Could you check a few things on this model? Use its own coordinates, in mm. A direction names the side the tool comes from. Coordinates: 2 decimals unless noted, no trailing zeros. Loops run counter-clockwise (first coordinate to the right, second up) from the corner with the lowest first, then second, coordinate; pieces in that order, holes last.
Autodesk Inventor part; units mm, degrees
ref_plane "Work Plane1" through (-19.708, -8.44, -77.2303) normal (0, 1, 0) x (0, 0, 1)
ref_plane "YZ Plane" through (0, 0, 0) normal (1, 0, 0) x (0, 1, 0)
ref_plane "XZ Plane" through (0, 0, 0) normal (0, 1, 0) x (-1, 0, 0)
sketch "Sketch1" plane through (0, 0, 0) normal (0, 1, 0) x (-1, 0, 0)
  line L0 (7.5, 17.125) -> (-7.5, 17.125)
  line L1 (-9.5, 15.125) -> (-9.5, -15.125)
  line L2 (-7.5, -17.125) -> (7.5, -17.125)
  line L3 (9.5, -15.125) -> (9.5, 15.125)
  line L4 (9.5, 17.125) -> (-9.5, -17.125) construction
  line L5 (-9.5, 17.125) -> (9.5, -17.125) construction
  arc A0 (7.5, -17.125) -> (9.5, -15.125) centre (7.5, -15.125) ccw
  arc A1 (-9.5, -15.125) -> (-7.5, -17.125) centre (-7.5, -15.125) ccw
  arc A2 (-7.5, 17.125) -> (-9.5, 15.125) centre (-7.5, 15.125) ccw
  arc A3 (9.5, 15.125) -> (7.5, 17.125) centre (7.5, 15.125) ccw
  point P0 (0, 0)
  dimension "d0" = 19
  dimension "d1" = 34.25
  dimension "d2" = 2
extrude "Extrusion1" add sketch "Sketch1" along normal blind 1.28
sketch "Sketch2" plane through (0, 1.28, 0) normal (0, 1, 0) x (1, 0, 0)
  line L0 (8.5, -12.175) -> (8.5, 15.825)
  line L1 (8.5, 15.825) -> (-8.5, 15.825)
  line L2 (-8.5, 15.825) -> (-8.5, -12.175)
  line L3 (-8.5, -12.175) -> (8.5, 15.825) construction
  line L4 (8.5, -12.175) -> (-8.5, 15.825) construction
  line L5 (7.5, 17.125) -> (-7.5, 17.125)
  line L6 (0, 17.125) -> (0, 15.825)
  line L7 (-6, -10.975) -> (6, -10.975)
  line L8 (6, -10.975) -> (6, -12.175)
  line L9 (-6, -12.175) -> (-6, -10.975)
  line L10 (-8.5, -12.175) -> (-6, -12.175)
  line L11 (6, -12.175) -> (8.5, -12.175)
  point P0 (0, 0)
  point P1 (0, 15.825)
  dimension "d5" = 17
  dimension "d6" = 28
  dimension "d7" = 1.3
  dimension "d9" = 1.2
extrude "Extrusion2" add sketch "Sketch2" along normal blind 1.28
sketch "Sketch3" plane through (0, 0, 0) normal (0, -1, 0) x (1, 0, 0)
  line L0 (5.75, -9.895) -> (-5.75, -9.895)
  line L1 (-5.75, -9.895) -> (-5.75, 6.605)
  line L2 (-5.75, 6.605) -> (5.75, 6.605)
  line L3 (5.75, 6.605) -> (5.75, -9.895)
  line L4 (7.5, -17.125) -> (-7.5, -17.125)
  line L5 (0, -17.125) -> (0, -9.895)
  point P0 (0, 0)
  point P1 (0, -9.895)
  dimension "d12" = 11.5
  dimension "d13" = 16.5
  dimension "d14" = 7.23
extrude "Extrusion3" add sketch "Sketch3" along normal blind 1.28
sketch "Sketch4" plane through (0, 0, 0) normal (0, -1, 0) x (1, 0, 0)
  line L0 (-7.5, 17.125) -> (7.5, 17.125)
  line L1 (0, 17.125) -> (0, 15.125)
  line L2 (0.2, 15.125) -> (2.24, 15.125)
  line L3 (2.44, 14.925) -> (2.44, 12.885)
  line L4 (2.24, 12.685) -> (0.2, 12.685)
  line L5 (0, 12.885) -> (0, 14.925)
  line L6 (0, 14.925) -> (0.2, 15.125)
  line L7 (2.24, 15.125) -> (2.44, 14.925)
  line L8 (2.44, 12.885) -> (2.24, 12.685)
  line L9 (0.2, 12.685) -> (0, 12.885)
  line L10 (2.64, 15.125) -> (4.68, 15.125)
  line L11 (4.88, 14.925) -> (4.88, 12.885)
  line L12 (4.68, 12.685) -> (2.64, 12.685)
  line L13 (2.44, 12.885) -> (2.44, 14.925)
  line L14 (2.44, 14.925) -> (2.64, 15.125)
  line L15 (4.68, 15.125) -> (4.88, 14.925)
  line L16 (4.88, 12.885) -> (4.68, 12.685)
  line L17 (2.64, 12.685) -> (2.44, 12.885)
  line L18 (5.08, 15.125) -> (7.12, 15.125)
  line L19 (7.32, 14.925) -> (7.32, 12.885)
  line L20 (7.12, 12.685) -> (5.08, 12.685)
  line L21 (4.88, 12.885) -> (4.88, 14.925)
  line L22 (4.88, 14.925) -> (5.08, 15.125)
  line L23 (7.12, 15.125) -> (7.32, 14.925)
  line L24 (7.32, 12.885) -> (7.12, 12.685)
  line L25 (5.08, 12.685) -> (4.88, 12.885)
  line L26 (-2.24, 15.125) -> (-0.2, 15.125)
  line L27 (0, 14.925) -> (0, 12.885)
  line L28 (-0.2, 12.685) -> (-2.24, 12.685)
  line L29 (-2.44, 12.885) -> (-2.44, 14.925)
  line L30 (-2.44, 14.925) -> (-2.24, 15.125)
  line L31 (-0.2, 15.125) -> (0, 14.925)
  line L32 (0, 12.885) -> (-0.2, 12.685)
  line L33 (-2.24, 12.685) -> (-2.44, 12.885)
  line L34 (-4.68, 15.125) -> (-2.64, 15.125)
  line L35 (-2.44, 14.925) -> (-2.44, 12.885)
  line L36 (-2.64, 12.685) -> (-4.68, 12.685)
  line L37 (-4.88, 12.885) -> (-4.88, 14.925)
  line L38 (-4.88, 14.925) -> (-4.68, 15.125)
  line L39 (-2.64, 15.125) -> (-2.44, 14.925)
  line L40 (-2.44, 12.885) -> (-2.64, 12.685)
  line L41 (-4.68, 12.685) -> (-4.88, 12.885)
  line L42 (-7.12, 15.125) -> (-5.08, 15.125)
  line L43 (-4.88, 14.925) -> (-4.88, 12.885)
  line L44 (-5.08, 12.685) -> (-7.12, 12.685)
  line L45 (-7.32, 12.885) -> (-7.32, 14.925)
  line L46 (-7.32, 14.925) -> (-7.12, 15.125)
  line L47 (-5.08, 15.125) -> (-4.88, 14.925)
  line L48 (-4.88, 12.885) -> (-5.08, 12.685)
  line L49 (-7.12, 12.685) -> (-7.32, 12.885)
  point P0 (0, 0)
  point P1 (2.44, 12.685)
  point P2 (2.44, 15.125)
  point P3 (0, 12.685)
  point P4 (2.44, 15.125)
  point P5 (4.88, 12.685)
  point P6 (4.88, 15.125)
  point P7 (2.44, 12.685)
  point P8 (4.88, 15.125)
  point P9 (7.32, 12.685)
  point P10 (7.32, 15.125)
  point P11 (4.88, 12.685)
  point P12 (-2.44, 15.125)
  point P13 (0, 12.685)
  point P14 (-2.44, 12.685)
  point P15 (-4.88, 15.125)
  point P16 (-2.44, 12.685)
  point P17 (-2.44, 15.125)
  point P18 (-4.88, 12.685)
  point P19 (-7.32, 15.125)
  point P20 (-4.88, 12.685)
  point P21 (-4.88, 15.125)
  point P22 (-7.32, 12.685)
  dimension "d27" = 2
extrude "Extrusion4" add sketch "Sketch4" along normal blind 2.44
sketch "Sketch5" plane through (0, -2.44, 0) normal (0, -1, 0) x (1, 0, 0)
  line L0 (-7.865, 15.055) -> (7.865, 15.055)
  line L1 (7.865, 15.055) -> (7.865, 12.755)
  line L2 (7.865, 12.755) -> (-7.865, 12.755)
  line L3 (-7.865, 12.755) -> (-7.865, 15.055)
  line L4 (0.2, 12.685) -> (0, 12.885)
  line L5 (0, 14.925) -> (0, 12.885)
  point P0 (0, 0)
  point P1 (0, 13.905)
  point P2 (0, 13.905)
  dimension "d30" = 15.73
  dimension "d31" = 2.3
extrude "Extrusion5" add sketch "Sketch5" along normal blind 6
sketch "Sketch6" plane through (0, 2.56, 0) normal (0, 1, 0) x (1, 0, 0)
  line L0 (-1.9361, 4.2441) -> (1.9639, 4.2441)
  line L1 (1.9639, 4.2441) -> (1.9639, 9.2441)
  line L2 (1.9639, 9.2441) -> (-1.9361, 9.2441)
  line L3 (-1.9361, 9.2441) -> (-1.9361, 4.2441)
  line L4 (-6.3946, -7.0839) -> (-2.0946, -7.0839)
  line L5 (-2.0946, -7.0839) -> (-2.0946, -3.9839)
  line L6 (-2.0946, -3.9839) -> (-6.3946, -3.9839)
  line L7 (-6.3946, -3.9839) -> (-6.3946, -7.0839)
  line L8 (3.9309, -7.1914) -> (5.5309, -7.1914)
  line L9 (5.5309, -7.1914) -> (5.5309, -4.1914)
  line L10 (5.5309, -4.1914) -> (3.9309, -4.1914)
  line L11 (3.9309, -4.1914) -> (3.9309, -7.1914)
  line L12 (8.5, 15.825) -> (-8.5, 15.825)
  point P0 (0, 0)
  point P1 (3.9309, -5.6914)
  point P2 (0, 15.825)
  point P3 (0.0139, 9.2441)
  point P4 (-2.0946, -5.5339)
  dimension "d34" = 3.9
  dimension "d35" = 5
  dimension "d36" = 4.3
  dimension "d37" = 3.1
  dimension "d38" = 1.6
  dimension "d39" = 3
extrude "Extrusion6" add sketch "Sketch6" along normal blind 1.5
sketch "Sketch7" plane through (0, -1.28, 0) normal (0, -1, 0) x (1, 0, 0)
  line L0 (-9, 11.5) -> (9, 11.5)
  line L1 (9, 11.5) -> (9, -11.5)
  line L2 (-8.5, -11.5) -> (-9, -11.5)
  line L3 (-9, -11.5) -> (-9, 11.5)
  line L4 (-9, -11.5) -> (-9, -15)
  line L5 (-8.5, -15.825) -> (-8.5, 12.175)
  line L6 (-9, -11.5) -> (-5.5, -11.5) construction
  line L7 (-9, -15) -> (9, -15)
  line L8 (9, -15) -> (9, -11.5)
  dimension "d42" = 18
  dimension "d43" = 23
  dimension "d46" = 3.5
  dimension "d47" = 90
  dimension "d48" = 90
ref_plane "Work Plane1" through (-19.708, -8.44, -77.2303) normal (0, 1, 0) x (0, 0, 1)
extrude "Extrusion7" add sketch "Sketch7" along normal up to surface (7.16 mm away)
properties part number "BMS"
(1) Imagine slicing it at C-C, the plane y = -4.5. Write out the boundary of the cut face in (x, z) (3 decimals).
Answers:
outline: (-9, -15) - (9, -15) - (9, 11.5) - (-9, 11.5) - close; (-7.865, 12.755) - (7.865, 12.755) - (7.865, 15.055) - (-7.865, 15.055) - close
(2) Which directions (+Z, -Z, +X, -X, +Y, -Y) give clear straight access to the entire face, cutting with the end or side of a thin tool? Please do faces 1 (the face through (5, 3, 7.191)), 2 (the face through (6, -1, 15.125)), 3 (the face through (-6, -1, 12.685)).
Answers:
face 1: +Z, +X, -X, +Y
face 2: +Z, +X, -X, -Y
face 3: +X, -X, -Y
(3) Imagine slicing it at A-A, the plane z = 10. Write out the boundary of the cut face in (x, y), and give its area (3 significant figures).
Answers:
outline: (-9.5, 0) - (9.5, 0) - (9.5, 1.28) - (8.5, 1.28) - (8.5, 2.56) - (-8.5, 2.56) - (-8.5, 1.28) - (-9.5, 1.28) - close; (-9, -8.44) - (9, -8.44) - (9, -1.28) - (-9, -1.28) - close
area: 175 mm2
(4) I need wall thicknesses on probe 1 along Z at (x, y) = (1.5, -4.25) (3 decimals); probe 2 along Y at (x, z) = (6.5, 6.5); probe 3 along X at (y, z) = (-2, -13.5). Which ranges of each line are inside material? Lowest first, please.
Answers:
probe 1: z = -15 to 11.5, 12.755 to 15.055
probe 2: y = -8.44 to -1.28, 0 to 2.56
probe 3: x = -9 to 9
(5) We'd pull the mould along Y, two halves only. Please class faces 4 (the face through (-4, 4.06, 6)), 5 (the face through (7.32, -1, 14)), 6 (the face through (4, -1, 15.125)): +Y half, -Y half, draft (parallel to the pull), parting line (faces both ways), or undercut.
Answers:
face 4: +Y half
face 5: undercut
face 6: draft
(6) Imagine slicing it at B-B, the plane x = -6.75. Write out the boundary of the cut face in (y, z) (3 decimals), and give its area (3 significant figures).
Answers:
outline: (-8.44, -15) - (-1.28, -15) - (-1.28, 11.5) - (-8.44, 11.5) - close; (-8.44, 12.755) - (-2.44, 12.755) - (-2.44, 12.685) - (0, 12.685) - (0, -17.125) - (1.28, -17.125) - (1.28, -15.825) - (2.56, -15.825) - (2.56, 12.175) - (1.28, 12.175) - (1.28, 17.125) - (0, 17.125) - (0, 15.125) - (-2.44, 15.125) - (-2.44, 15.055) - (-8.44, 15.055) - close
area: 289 mm2
(7) Imagine slicing it at D-D, the plane z = 14. Write out the boundary of the cut face in (x, y) (3 decimals), and give its area (3 significant figures).
Answers:
outline: (-9.5, 0) - (-7.32, 0) - (-7.32, -2.44) - (-7.865, -2.44) - (-7.865, -8.44) - (7.865, -8.44) - (7.865, -2.44) - (7.32, -2.44) - (7.32, 0) - (9.5, 0) - (9.5, 1.28) - (-9.5, 1.28) - close
area: 154 mm2
(8) For pin 1 (1 mm diameter, centred on x = 2, y = -1.5, fed in from -Z); pin 2 (9 mm diameter, centred on x = -1.5, z = -3.5, fed in from +Y); pin 3 (2 mm diameter, centred on x = 3, y = 2.5, fed in from +Z) (3 decimals); pin 4 (2 mm diameter, centred on y = -3, z = 10.5, fed in from +X), each with a flat end and sliding along its axis, tell me the tip position at first contact or that it passes through.
Answers:
pin 1: stops at z = -15
pin 2: stops at y = 4.06
pin 3: stops at z = 10.975
pin 4: stops at x = 9
